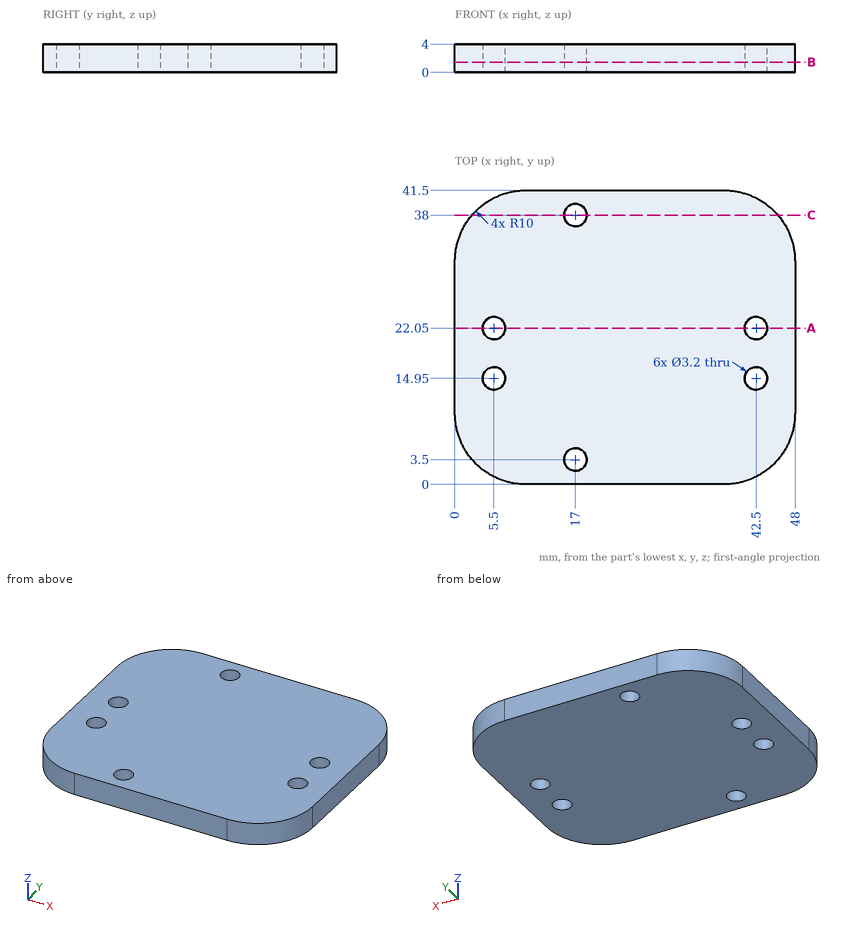
Here's the drawing with two shaded views (mm, measured from the low corner). I have some questions. Round coordinates to 2 decimals unless told otherwise and drop trailing zeros. Order: outer loops, then holes, each group sorted by start corner. A loop starts at its lowest first (then second) coordinate and runs counter-clockwise, first axis right, second up. Notation, with made-up numbers: (18.5, 56.5) -> (54.5, 56.5) arc R23 cw to (54.5, 87.5) -> close; hole circle Ø4 at (-30.5, 44). An arc over 180 degrees is marked (long way). Return JSON: item names as keys, results as strings.
Q1. If we section it at A-A on y = 22.05: List the corners of the cut face in (x, z) for me, plus the area to 3 significant figures.
Filled sheet:
{"outline": "(0, 0) -> (3.9, 0) -> (3.9, 4) -> (0, 4) -> close; (7.1, 0) -> (40.9, 0) -> (40.9, 4) -> (7.1, 4) -> close; (44.1, 0) -> (48, 0) -> (48, 4) -> (44.1, 4) -> close", "area": "166 mm^2"}
Q2. For pin 1 Ø2 at (y, z) = (5, 1) entering from +X, with a flat end and sliding along its axis, tell me the tip position at first contact or that it passes through.
Filled sheet:
{"pin 1": "stops at x = 47.17"}
Q3. If we section it at C-C on y = 38: List the corners of the cut face in (x, z) for me, plus the area to 3 significant figures.
Filled sheet:
{"outline": "(2.4, 0) -> (15.4, 0) -> (15.4, 4) -> (2.4, 4) -> close; (18.6, 0) -> (45.6, 0) -> (45.6, 4) -> (18.6, 4) -> close", "area": "160 mm^2"}
Q4. I need wall thicknesses on line 1 along X through (y, z) = (22.05, 1.6); line 2 along Y through (x, z) = (17, 2.95); line 3 along Y through (x, z) = (42.5, 1.95). Which ranges of each line are inside material? Lowest first, please. Write a range as from..to.
Filled sheet:
{"line 1": "x = 0..3.9, 7.1..40.9, 44.1..48", "line 2": "y = 0..1.9, 5.1..36.4, 39.6..41.5", "line 3": "y = 1.07..13.35, 16.55..20.45, 23.65..40.43"}
Q5. If we section it at B-B on z = 1.45: List the corners of the cut face in (x, y) for me, plus the area to 3 significant figures.
Filled sheet:
{"outline": "(0, 10) arc R10 ccw to (10, 0) -> (38, 0) arc R10 ccw to (48, 10) -> (48, 31.5) arc R10 ccw to (38, 41.5) -> (10, 41.5) arc R10 ccw to (0, 31.5) -> close; hole circle Ø3.2 at (5.5, 14.95); hole circle Ø3.2 at (5.5, 22.05); hole circle Ø3.2 at (17, 3.5); hole circle Ø3.2 at (17, 38); hole circle Ø3.2 at (42.5, 14.95); hole circle Ø3.2 at (42.5, 22.05)", "area": "1,860 mm^2"}
